Here's how the part is built. I have some questions about the finished solid (model axes, mm). Face numbers are marked on the shaded views. A direction names the side the tool comes from. Give positions to 0.01 mm unless a question says otherwise; leave off trailing zeros. Order: outer loops, then holes, each group sorted by start corner. A loop starts at its lowest first (then second) coordinate and runs counter-clockwise, first axis right, second up. Notation, with made-up numbers: (-27, 24) -> (14, 24) arc R27 ccw to (14, 43) -> close; hole circle Ø7 at (-16.5, -5). An arc over 180 degrees is marked (long way). Write each question's results on one line, items separated by ' | '. Start each with the question number.
Q1. Imagine slicing it at D-D, the plane x = -7. Please give me the cut outline in (y, z) (3 decimals), then the cut area to 3 significant figures.
Q2. For the marked faces 1, 2, 3 and 4, which set-ups out of +Z, -Z, +X, -X, +Y, -Y let a thin tool reach every point of the face, with its end or its side?
Q3. I need wall thicknesses on line 1 along X through (y, z) = (4.6, 0); line 2 along X through (y, z) = (5.5, 4.75); line 3 along X through (y, z) = (-5.25, 3.5). Which ranges of each line are inside material? Lowest first, please. Write a range as [from, to].
Q4. Imagine slicing it at B-B, the plane x = 2. Please give me the cut outline in (y, z) (3 decimals).
Q5. I'm going to push flat-ended pins straight in: pin 1 (2 mm diameter, centred on x = 6, y = 5, fed in from +Z); pin 2 (1 mm diameter, centred on x = 5.5, z = -8, fed in from +Y); pin 3 (1.9 mm diameter, centred on x = 4.9, z = 0, fed in from -Y); pin 4 (11.5 mm diameter, centred on y = 1, z = -2, fed in from -X). Where does each tip first touch, or does it pass through?
Q6. Thinking about a two-plate mould opening in Y: for the marked faces 5, 6 and 7, which applies, pulls with the +Y half, pulls with the -Y half, needs draft (parallel to the pull), parting line crosses it, or undercut?
Q7. Imagine slicing it at A-A, the plane y = 0. State how many separate pieces and enclosed holes the cut face has, then the cut area to 3 significant figures.
```python
from build123d import *

# Parameters (mm, degrees)
SKETCH3_R         = 1.0287
SCREW_HOLE_DEPTH  = 11.033
CIRPATTERN1_COUNT = 2
CIRPATTERN1_ANGLE = 90
FILLET1_R         = 0.381


with BuildPart() as part:
    # Sketch2 → PULLEY (revolve)
    with BuildSketch(Plane.XY):
        Polygon((-8.6725125, 3.175), (8.6725125, 3.175), (8.6725125, 5.6134), (1.1318875, 5.6134), (1.1318875, 7.23646), (0.1514475, 7.23646), (0.1514475, 8.2169), (-7.6920725, 8.2169), (-7.6920725, 7.23646), (-8.6725125, 7.23646), align=None)
    revolve(axis=Axis((-8.6725125, 0, 0), (1, 0, 0)))

    # Sketch4 → Flange (revolve)
    with BuildSketch(Plane.XY):
        Polygon((-8.1822925, 7.23646), (-8.1822925, 8.2169), (-8.7899875, 10.033), (-8.2997675, 10.033), (-7.6920725, 8.2169), (-7.6920725, 7.23646), align=None)
        Polygon((0.1514475, 7.23646), (0.6416675, 7.23646), (0.6416675, 8.2169), (1.2493625, 10.033), (0.7591425, 10.033), (0.1514475, 8.2169), align=None)
    revolve(axis=Axis((0, 0, 0), (-1, 0, 0)))

    # Sketch3 → SCREW HOLE (cut, through all)
    with BuildSketch(Plane(origin=(0, 0, 0), x_dir=(1, 0, 0), z_dir=(0, 1, 0))):
        with Locations((4.9022, 0)):
            Circle(SKETCH3_R)
    screw_hole = extrude(amount=SCREW_HOLE_DEPTH, mode=Mode.SUBTRACT)

    # CirPattern1: SCREW HOLE ×2 about axis
    cirpattern1_axis = Axis((-8.6725125, 0, 0), (-1, 0, 0))
    for i in range(1, CIRPATTERN1_COUNT):
        add(screw_hole.rotate(cirpattern1_axis, i * CIRPATTERN1_ANGLE / (CIRPATTERN1_COUNT - 1)), mode=Mode.SUBTRACT)

    # Fillet1
    fillet1_edges = [part.edges().sort_by_distance(p)[0] for p in [
        (-8.6725125, -3.175, 0),
        (8.6725125, -3.175, 0),
        (8.6725125, -5.6134, 0),
    ]]
    fillet(fillet1_edges, radius=FILLET1_R)


solid = part.part
```
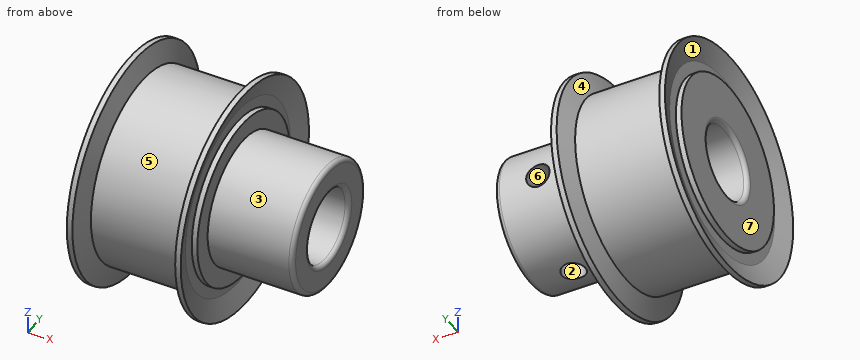
Geometry check:
1) outline: circle Ø16.434 at (0, 0); hole circle Ø6.35 at (0, 0) | area: 180 mm²
2) face 1: -X | face 2: -Z | face 3: +X | face 4: none
3) line 1: [-8.67, 3.87], [5.93, 8.67] | line 2: [-8.18, 0.64] | line 3: [-8.67, 1.13]
4) outline: circle Ø11.227 at (0, 0); hole circle Ø6.35 at (0, 0)
5) pin 1: z = 3.94 | pin 2: through | pin 3: y = -5.61 | pin 4: x = -8.67
6) face 5: parting line crosses it | face 6: needs draft | face 7: undercut
7) separate pieces: 3 | enclosed holes: 0 | area: 132 mm²
